Could you check a few things on this model? Use its own coordinates, in mm. Face numbers are marked on the shaded views. A direction names the side the tool comes from. Coordinates: 2 decimals unless noted, no trailing zeros. Order: outer loops, then holes, each group sorted by start corner. A loop starts at its lowest first (then second) coordinate and runs counter-clockwise, first axis right, second up.
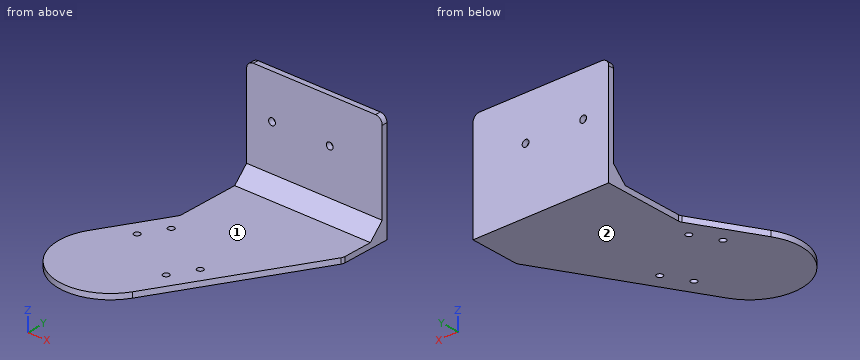
```python
from build123d import *

# Parameters (mm, degrees)
BOSS_EXTRUDE1_DEPTH = 8
SKETCH4_W           = 150
SKETCH4_H           = 8
BOSS_EXTRUDE2_DEPTH = 200
CHAMFER1_SIZE       = 20
CUT_EXTRUDE1_REACH  = 327
SKETCH5_R           = 5
CUT_EXTRUDE2_REACH  = 10
SKETCH6_R           = 4.5
FILLET1_R           = 10


with BuildPart() as part:
    # Sketch1 → Boss-Extrude1 (new body)
    with BuildSketch(Plane.XY):
        with BuildLine():
            Line((-64.951905284, 37.5), (-11.547005384, 130))
            Line((-11.547005384, 130), (-11.547005384, 250))
            Line((-11.547005384, 250), (188.452994616, 250))
            Line((188.452994616, 250), (188.452994616, 176.410161514))
            Line((188.452994616, 176.410161514), (64.951905284, -37.5))
            ThreePointArc((64.951905284, -37.5), (-37.5, -64.951905284), (-64.951905284, 37.5))
        make_face()
    extrude(amount=BOSS_EXTRUDE1_DEPTH)

    # Sketch4 → Boss-Extrude2 (add)
    with BuildSketch(Plane.ZY.offset(11.547005384)):
        with Locations((83, 246)):
            Rectangle(SKETCH4_W, SKETCH4_H)
    extrude(amount=-BOSS_EXTRUDE2_DEPTH)

    # Chamfer1
    chamfer1_edges = [part.edges().sort_by_distance(p)[0] for p in [
        (88.452994616, 242, 8),
    ]]
    chamfer(chamfer1_edges, length=CHAMFER1_SIZE)

    # Sketch5 → Cut-Extrude1 (cut, up to next)
    with BuildSketch(Plane(origin=(0, 250, 0), x_dir=(1, 0, 0), z_dir=(0, 1, 0)), mode=Mode.PRIVATE) as cut_extrude1_sk1:
        with Locations((25.952994616, -94)):
            Circle(SKETCH5_R)
    cut_extrude1_tool1 = extrude(cut_extrude1_sk1.sketch, amount=-CUT_EXTRUDE1_REACH, mode=Mode.PRIVATE) & part.part
    add(cut_extrude1_tool1.solids().sort_by_distance((25.952995, 250, 94))[0], mode=Mode.SUBTRACT)
    # Sketch5 → Cut-Extrude1 (cut, up to next)
    with BuildSketch(Plane(origin=(0, 250, 0), x_dir=(1, 0, 0), z_dir=(0, 1, 0)), mode=Mode.PRIVATE) as cut_extrude1_sk2:
        with Locations((110.952994616, -94)):
            Circle(SKETCH5_R)
    cut_extrude1_tool2 = extrude(cut_extrude1_sk2.sketch, amount=-CUT_EXTRUDE1_REACH, mode=Mode.PRIVATE) & part.part
    add(cut_extrude1_tool2.solids().sort_by_distance((110.952995, 250, 94))[0], mode=Mode.SUBTRACT)

    # Sketch6 → Cut-Extrude2 (cut, up to next)
    with BuildSketch(Plane.XY.offset(8), mode=Mode.PRIVATE) as cut_extrude2_sk1:
        with Locations((0.698729811, 101.210235533)):
            Circle(SKETCH6_R)
    cut_extrude2_tool1 = extrude(cut_extrude2_sk1.sketch, amount=-CUT_EXTRUDE2_REACH, mode=Mode.PRIVATE) & part.part
    add(cut_extrude2_tool1.solids().sort_by_distance((0.69873, 101.210236, 8))[0], mode=Mode.SUBTRACT)
    # Sketch6 → Cut-Extrude2 (cut, up to next)
    with BuildSketch(Plane.XY.offset(8), mode=Mode.PRIVATE) as cut_extrude2_sk2:
        with Locations((87.301270189, 51.210235533)):
            Circle(SKETCH6_R)
    cut_extrude2_tool2 = extrude(cut_extrude2_sk2.sketch, amount=-CUT_EXTRUDE2_REACH, mode=Mode.PRIVATE) & part.part
    add(cut_extrude2_tool2.solids().sort_by_distance((87.30127, 51.210236, 8))[0], mode=Mode.SUBTRACT)
    # Sketch6 → Cut-Extrude2 (cut, up to next)
    with BuildSketch(Plane.XY.offset(8), mode=Mode.PRIVATE) as cut_extrude2_sk3:
        with Locations((67.301270189, 16.569219382)):
            Circle(SKETCH6_R)
    cut_extrude2_tool3 = extrude(cut_extrude2_sk3.sketch, amount=-CUT_EXTRUDE2_REACH, mode=Mode.PRIVATE) & part.part
    add(cut_extrude2_tool3.solids().sort_by_distance((67.30127, 16.569219, 8))[0], mode=Mode.SUBTRACT)
    # Sketch6 → Cut-Extrude2 (cut, up to next)
    with BuildSketch(Plane.XY.offset(8), mode=Mode.PRIVATE) as cut_extrude2_sk4:
        with Locations((-19.301270189, 66.569219382)):
            Circle(SKETCH6_R)
    cut_extrude2_tool4 = extrude(cut_extrude2_sk4.sketch, amount=-CUT_EXTRUDE2_REACH, mode=Mode.PRIVATE) & part.part
    add(cut_extrude2_tool4.solids().sort_by_distance((-19.30127, 66.569219, 8))[0], mode=Mode.SUBTRACT)

    # Fillet1
    fillet1_edges = [part.edges().sort_by_distance(p)[0] for p in [
        (-11.547005384, 130, 4),
        (188.452994616, 176.410161514, 4),
        (188.452994616, 246, 158),
        (-11.547005384, 246, 158),
    ]]
    fillet(fillet1_edges, radius=FILLET1_R)


solid = part.part
```
Item 1: Suppose I cut it at B-B (x = 97). List the corners of the cut face in (y, z) for me.
Item 2: For pin 1 Ø13 at (x, z) = (25.95, 94) entering from -Y; pin 2 Ø8 at (x, z) = (110.95, 94) entering from -Y; pin 3 Ø10 at (x, z) = (80, 25.5) entering from -Y; pin 4 Ø2 at (x, y) = (-24, 56) entering from +Z, each with a flat end and sliding along its axis, tell me the tip position at first contact or that it passes through.
Item 3: Suppose I cut it at D-D (y = 155). List the corners of the cut face in (x, z) for me.
Item 4: Which directions (+Z, -Z, +X, -X, +Y, -Y) give clear straight access to the entire face, cutting with the end or side of a thin tool? Please do the marked faces 1 and 2.
Item 5: Suppose I cut it at C-C (z = 22). List the corners of the cut face in (x, y) for me, and give its area (3 significant figures).
Item 6: Suppose I cut it at A-A (z = 94). List the corners of the cut face in (x, y) for me.
Item 7: I need wall thicknesses on line 1 (X direction, y = 247, z = 94); line 2 (Y direction, x = 91, z = 97); line 3 (Z direction, x = 65, y = 116.5). Which ranges of each line are inside material? Lowest first, please.
Geometry results:
1. outline: (18.01, 0) - (250, 0) - (250, 158) - (242, 158) - (242, 28) - (222, 8) - (18.01, 8) - close
2. pin 1: stops at y = 242
2. pin 2: passes through
2. pin 3: stops at y = 234.5
2. pin 4: stops at z = 8
3. outline: (-11.55, 0) - (176.09, 0) - (176.09, 8) - (-11.55, 8) - close
4. face 1: +Z, +X, -X, -Y
4. face 2: -Z, +X, -X, +Y, -Y
5. outline: (-11.55, 236) - (188.45, 236) - (188.45, 250) - (-11.55, 250) - close
5. area: 2,800 mm2
6. outline: (-11.55, 242) - (20.95, 242) - (20.95, 250) - (-11.55, 250) - close; (30.95, 242) - (105.95, 242) - (105.95, 250) - (30.95, 250) - close; (115.95, 242) - (188.45, 242) - (188.45, 250) - (115.95, 250) - close
7. line 1: x = -11.55 to 20.95, 30.95 to 105.95, 115.95 to 188.45
7. line 2: y = 242 to 250
7. line 3: z = 0 to 8
